Answer from the drawing. Dimensions are ordinates in mm from the lowest x, y and z of the part. Give positions to 0.01 mm unless a question says otherwise; leave off trailing zeros. Order: outer loops, then holes, each group sorted by start corner. A loop starts at its lowest first (then second) coordinate and runs counter-clockwise, first axis right, second up. Notation, with made-up numbers: M -16.75,47 L 11.25,47 A24 cw 11.25,71 Z; hole C -36.75,58 d5. An arc over 180 degrees is marked long. One line per item, written item: value.
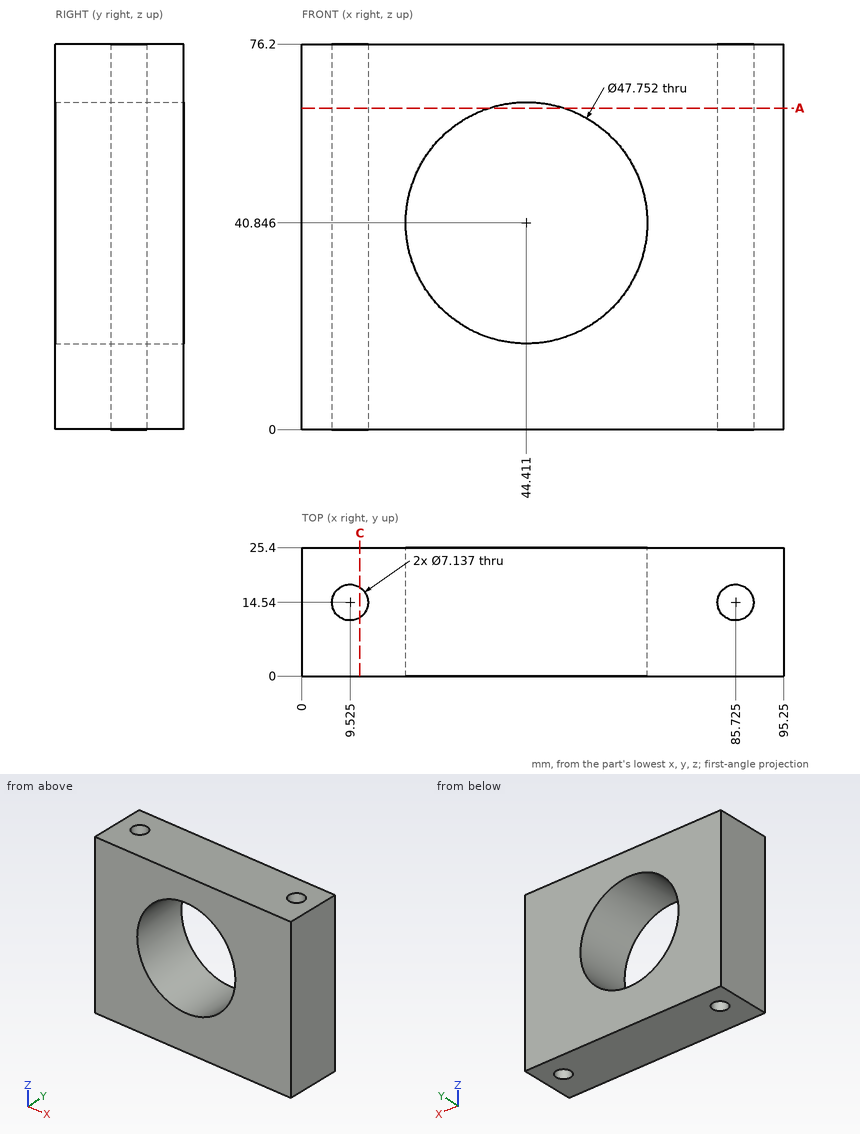
(1) Find the intervals of material crossed by probe 1 along Z at (x, y) = (58.5, 2.75); probe 2 along X at (y, z) = (15.75, 67); probe 3 along X at (y, z) = (9.5, 33), in increasing order. Write a range as from..to.
Findings:
probe 1: z = 0..21.57, 60.12..76.2
probe 2: x = 0..6.17, 12.88..82.37, 89.08..95.25
probe 3: x = 0..21.86, 66.96..95.25
(2) Section A-A, the plane z = 63.5 is taken. Give the number of separate pieces and of enclosed holes in the cut face, then the cut area to 3 significant figures.
Findings:
separate pieces: 2
enclosed holes: 2
area: 1,960 mm^2
(3) Section C-C, the plane x = 11.5 is taken. Give the vertices of the cut face in (y, z).
Findings:
outline: M 0,0 L 11.57,0 L 11.57,76.2 L 0,76.2 Z; M 17.51,0 L 25.4,0 L 25.4,76.2 L 17.51,76.2 Z
